Can you work these out from the model? Positions are in its coordinate system, mm. A direction names the side the tool comes from. Coordinates: 2 decimals unless noted, no trailing zeros. Order: outer loops, then holes, each group sorted by start corner. A loop starts at its lowest first (then second) coordinate and runs counter-clockwise, first axis right, second up. Notation, with made-up numbers: (-27.75, 13) -> (13.25, 13) arc R9 cw to (13.25, 18) -> close; hole circle Ø5 at (6.25, 44). An arc over 180 degrees is marked (long way). Answer as CSV lines item,"result".
from build123d import *

# Parameters (mm, degrees)
SKETCH_1_W          = 32
SKETCH_1_H          = 69.6
EXTRUDE_1_DEPTH     = 23
SKETCH_2_R          = 1.5
EXTRUDE_2_DEPTH     = 45.9
SKETCH_3_W          = 2
SKETCH_3_H          = 3.6
EXTRUDE_3_DEPTH     = 4.5
SKETCH_5_W          = 16
SKETCH_5_H          = 23
CUT_EXTRUDE_1_DEPTH = 71.5
SKETCH_6_W          = 4.5
SKETCH_6_H          = 3.6
CUT_EXTRUDE_2_DEPTH = 1
SKETCH_7_W          = 2
SKETCH_7_H          = 4.4
EXTRUDE_4_DEPTH     = 6.5
SKETCH_9_W          = 1
SKETCH_9_H          = 1.8
CUT_EXTRUDE_3_DEPTH = 4.5
SKETCH_10_W         = 1.5
SKETCH_10_H         = 2
EXTRUDE_5_DEPTH     = 4.5
SKETCH_12_W         = 2
SKETCH_12_H         = 4.395113111
EXTRUDE_6_DEPTH     = 7.5
SKETCH_15_W         = 2
SKETCH_15_H         = 3.6
EXTRUDE_7_DEPTH     = 6
SKETCH_14_R         = 1.801767182
CUT_EXTRUDE_4_DEPTH = 6
SKETCH_17_W         = 2
SKETCH_17_H         = 4.5
EXTRUDE_8_DEPTH     = 6
SKETCH_16_R         = 1.798109405
CUT_EXTRUDE_5_DEPTH = 6
SKETCH_18_R         = 1.5
CUT_EXTRUDE_6_DEPTH = 45.9


with BuildPart() as part:
    # ｽｹｯﾁ1 → ﾎﾞｽ - 押し出し1 (new body)
    with BuildSketch(Plane.XY):
        with Locations((50.279062003, -5.527058824)):
            Rectangle(SKETCH_1_W, SKETCH_1_H)
    extrude_1 = extrude(amount=EXTRUDE_1_DEPTH)

    # ｽｹｯﾁ2 → ﾎﾞｽ - 押し出し2 (add)
    with BuildSketch(Plane(origin=(66.279062003, 0, 0), x_dir=(0, 0, -1), z_dir=(1, 0, 0))):
        with Locations((-11.5, -27.627058824)):
            Circle(SKETCH_2_R)
    extrude_2 = extrude(amount=EXTRUDE_2_DEPTH)

    # ｽｹｯﾁ3 → ﾎﾞｽ - 押し出し3 (add)
    with BuildSketch(Plane(origin=(66.279062003, 0, 0), x_dir=(0, 0, -1), z_dir=(1, 0, 0))):
        with Locations((-1, -21.322089651)):
            Rectangle(SKETCH_3_W, SKETCH_3_H)
    extrude(amount=EXTRUDE_3_DEPTH)

    # ｽｹｯﾁ5 → ｶｯﾄ - 押し出し1 (cut)
    with BuildSketch(Plane(origin=(0, 29.272941176, 0), x_dir=(1, 0, 0), z_dir=(0, 1, 0))):
        with Locations((42.279062003, -11.5)):
            Rectangle(SKETCH_5_W, SKETCH_5_H)
    extrude(amount=-CUT_EXTRUDE_1_DEPTH, mode=Mode.SUBTRACT)

    # ｽｹｯﾁ6 → ｶｯﾄ - 押し出し2 (cut)
    with BuildSketch(Plane.XY.offset(2)):
        with Locations((68.529062003, -21.322089651)):
            Rectangle(SKETCH_6_W, SKETCH_6_H)
    extrude(amount=-CUT_EXTRUDE_2_DEPTH, mode=Mode.SUBTRACT)

    # ｽｹｯﾁ7 → ﾎﾞｽ - 押し出し4 (add)
    with BuildSketch(Plane(origin=(66.279062003, 0, 0), x_dir=(0, 0, -1), z_dir=(1, 0, 0))):
        with Locations((-1, -17.322089651)):
            Rectangle(SKETCH_7_W, SKETCH_7_H)
    extrude_4 = extrude(amount=EXTRUDE_4_DEPTH)

    # ｽｹｯﾁ9 → ｶｯﾄ - 押し出し3 (cut)
    with BuildSketch(Plane(origin=(70.779062003, 0, 0), x_dir=(0, 0, -1), z_dir=(1, 0, 0))):
        with Locations((-0.5, -22.222089651)):
            Rectangle(SKETCH_9_W, SKETCH_9_H)
    cut_extrude_3 = extrude(amount=-CUT_EXTRUDE_3_DEPTH, mode=Mode.SUBTRACT)

    # ﾐﾗｰ4: ﾎﾞｽ - 押し出し4, ｶｯﾄ - 押し出し3 across plane
    add(extrude_4.mirror(Plane(origin=(66.279062003, -21.322089651, 1), x_dir=(0, 0, 1), z_dir=(0, 1, 0))))
    add(cut_extrude_3.mirror(Plane(origin=(66.279062003, -21.322089651, 1), x_dir=(0, 0, 1), z_dir=(0, 1, 0))), mode=Mode.SUBTRACT)

    # ｽｹｯﾁ10 → ﾎﾞｽ - 押し出し5 (add)
    with BuildSketch(Plane.XZ.offset(19.522089651)):
        with Locations((72.029062003, 1)):
            Rectangle(SKETCH_10_W, SKETCH_10_H)
    extrude_5 = extrude(amount=EXTRUDE_5_DEPTH)

    # ﾐﾗｰ25: ﾎﾞｽ - 押し出し1, ﾎﾞｽ - 押し出し2, ﾎﾞｽ - 押し出し4, ﾎﾞｽ - 押し出し5 across plane
    add(extrude_1.mirror(Plane(origin=(50.279062003, -42.227058824, 0), x_dir=(0, 0, 1), z_dir=(1, 0, 0))))
    add(extrude_2.mirror(Plane(origin=(50.279062003, -42.227058824, 0), x_dir=(0, 0, 1), z_dir=(1, 0, 0))))
    add(extrude_4.mirror(Plane(origin=(50.279062003, -42.227058824, 0), x_dir=(0, 0, 1), z_dir=(1, 0, 0))))
    add(extrude_5.mirror(Plane(origin=(50.279062003, -42.227058824, 0), x_dir=(0, 0, 1), z_dir=(1, 0, 0))))

    # ｽｹｯﾁ12 → ﾎﾞｽ - 押し出し6 (add)
    with BuildSketch(Plane.ZY.offset(-27.779062003)):
        with Locations((1, -26.219646207)):
            Rectangle(SKETCH_12_W, SKETCH_12_H)
    extrude(amount=-EXTRUDE_6_DEPTH)

    # ｽｹｯﾁ15 → ﾎﾞｽ - 押し出し7 (add)
    with BuildSketch(Plane(origin=(66.279062003, 0, 0), x_dir=(0, 0, -1), z_dir=(1, 0, 0))):
        with Locations((-1, -21.322089651)):
            Rectangle(SKETCH_15_W, SKETCH_15_H)
    extrude(amount=EXTRUDE_7_DEPTH)

    # ｽｹｯﾁ14 → ｶｯﾄ - 押し出し4 (cut)
    with BuildSketch(Plane.XY.offset(2)):
        with Locations((69.477294821, -21.322089651)):
            Circle(SKETCH_14_R)
    extrude(amount=-CUT_EXTRUDE_4_DEPTH, mode=Mode.SUBTRACT)

    # ｽｹｯﾁ17 → ﾎﾞｽ - 押し出し8 (add)
    with BuildSketch(Plane.ZY.offset(-34.279062003)):
        with Locations((1, -21.772089651)):
            Rectangle(SKETCH_17_W, SKETCH_17_H)
    extrude(amount=EXTRUDE_8_DEPTH)

    # ｽｹｯﾁ16 → ｶｯﾄ - 押し出し5 (cut)
    with BuildSketch(Plane.XY.offset(2)):
        with Locations((31.077171408, -21.772089651)):
            Circle(SKETCH_16_R)
    extrude(amount=-CUT_EXTRUDE_5_DEPTH, mode=Mode.SUBTRACT)

    # ｽｹｯﾁ18 → ｶｯﾄ - 押し出し6 (cut)
    with BuildSketch(Plane.ZY.offset(11.620937997)):
        with Locations((11.5, -27.627058824)):
            Circle(SKETCH_18_R)
    extrude(amount=-CUT_EXTRUDE_6_DEPTH, mode=Mode.SUBTRACT)


solid = part.part
Q1. If I drill on line 1 (X direction, y = -24, z = 4.25), over which ranges is the centre line in solid material (lowest first)?
Solution:
line 1,"34.28 to 66.28"
Q2. For P1, Ø1, axis at x = 71, z = 0.5, coming from the +Y side; P2, Ø5, axis at x = 32, y = -25, coming from the +Z side; P3, Ø8, axis at y = -18.5, z = 7, coming from the +X side; P4, Ø1, axis at y = -21.5, z = 0.5, coming from the +X side, each with a flat end and sliding along its axis, tell me the tip position at first contact or that it passes through.
Solution:
P1,"y = -15.12"
P2,"z = 23"
P3,"x = 66.28"
P4,"x = 72.78"
Q3. Imagine slicing it at C-C (x = 101). List the corners of the cut face in (y, z) for me.
Solution:
outline,"circle Ø3 at (-27.63, 11.5)"
Q4. Imagine slicing it at A-A (z = 11.5). List the corners of the cut face in (x, y) for me, and give its area (3 significant figures).
Solution:
outline,"(34.28, -40.33) -> (66.28, -40.33) -> (66.28, -29.13) -> (112.18, -29.13) -> (112.18, -26.13) -> (66.28, -26.13) -> (66.28, 29.27) -> (34.28, 29.27) -> close"
area,"2,360 mm2"
Q5. Imagine slicing it at B-B (y = 19.5). List the corners of the cut face in (x, z) for me.
Solution:
outline,"(34.28, 0) -> (66.28, 0) -> (66.28, 23) -> (34.28, 23) -> close"
Q6. Which directions (+Z, -Z, +X, -X, +Y, -Y) give clear straight access to the entire face, cutting with the end or side of a thin tool? Please do faces 1 (the flat face through (71, -23, 2)), 2 (the flat face through (69, -27.522, 1)), 3 (the cylindrical face through (88.908, -26.613, 12.606)), 4 (the flat face through (69, -15.122, 1)), 5 (the flat face through (29.5, -23.3, 2)).
Solution:
face 1,"+X, +Y, -Y"
face 2,"-Z, +X, -Y"
face 3,"+X"
face 4,"+Z, -Z, +X, +Y"
face 5,"+Z, -X, +Y, -Y"
Q7. We'd pull the mould along Y, two halves only. Please class faces 6 (the flat face through (31, -15.122, 1)), 7 (the flat face through (31, -28.417, 1)), 8 (the cylindrical face through (29.28, -21.69, 1.01)): pulls with the +Y half, pulls with the -Y half, needs draft (parallel to the pull), parting line crosses it, or undercut.
Solution:
face 6,"pulls with the +Y half"
face 7,"pulls with the -Y half"
face 8,"undercut"
Q8. Imagine slicing it at D-D (z = 21.75). List the corners of the cut face in (x, y) for me, and give its area (3 significant figures).
Solution:
outline,"(34.28, -40.33) -> (66.28, -40.33) -> (66.28, 29.27) -> (34.28, 29.27) -> close"
area,"2,230 mm2"
